Verification items for the finished model (mm, model axes). Give positions to 0.01 mm unless a question says otherwise; leave off trailing zeros. Loops run counter-clockwise (first coordinate to the right, second up) from the corner with the lowest first, then second, coordinate; pieces in that order, holes last. Notation, with made-up numbers: M 24,-25 L 51,-25 A19 ccw 51,-8 Z; hole C -25.5,88.5 d5. An arc over 180 degrees is marked long. Answer in a Markdown table with one row per item.
```python
from build123d import *

# Parameters (mm, degrees)
SKETCH1_W               = 10
SKETCH1_H               = 10
SKETCH1_R               = 2.605
BOSS_EXTRUDE1_DEPTH     = 304.8
CIRPATTERN1_COUNT       = 4
SKETCH2_R               = 6.35
CUT_EXTRUDE1_DEPTH      = 20
CUT_EXTRUDE1_DEPTH_BACK = 30


with BuildPart() as part:
    # Sketch1 → Boss-Extrude1 (new body)
    with BuildSketch(Plane(origin=(0, 0, 0), x_dir=(0, 0, -1), z_dir=(1, 0, 0))):
        Rectangle(SKETCH1_W, SKETCH1_H)
        Circle(SKETCH1_R, mode=Mode.SUBTRACT)
        Polygon((7.474873734, 9.921463197), (2.553410537, 5), (5, 5), (5, 3.203948776), (9.596194078, 7.800142853), align=None)
        Polygon((9.596194078, 3.24), (12.596194078, 3.24), (12.596194078, 12.596194078), (3.24, 12.596194078), (3.24, 9.921463197), (7.474873734, 9.921463197), (9.596194078, 7.800142853), align=None)
    boss_extrude1 = extrude(amount=BOSS_EXTRUDE1_DEPTH)

    # CirPattern1: Boss-Extrude1 ×4 about axis
    cirpattern1_axis = Axis((0, 0, 0), (1, 0, 0))
    for i in range(1, CIRPATTERN1_COUNT):
        add(boss_extrude1.rotate(cirpattern1_axis, i * 360 / CIRPATTERN1_COUNT))

    # Sketch2 → Cut-Extrude1 (cut, two sides)
    with BuildSketch(Plane.XY) as cut_extrude1_sk:
        with Locations((152.4, 0)):
            Circle(SKETCH2_R)
    extrude(amount=CUT_EXTRUDE1_DEPTH, mode=Mode.SUBTRACT)
    extrude(cut_extrude1_sk.sketch, amount=-CUT_EXTRUDE1_DEPTH_BACK, mode=Mode.SUBTRACT)


solid = part.part
```
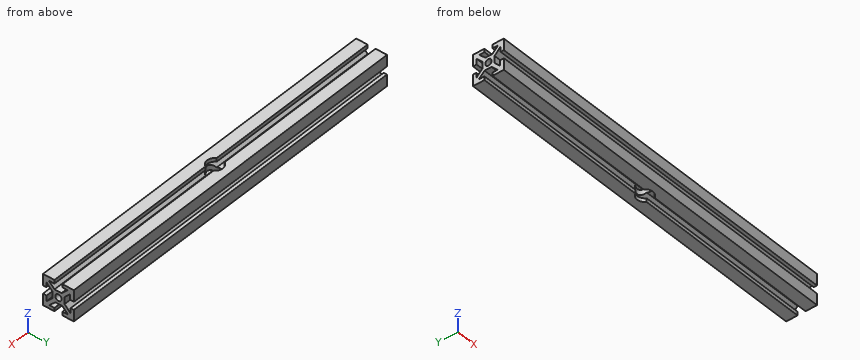
Item 1: Go/stop test with flat-tipped pins: pin 1 (3 mm diameter, centred on x = 103, y = -1.5, fed in from +Z); pin 2 (4.5 mm diameter, centred on x = 88, z = -0.5, fed in from -Y); pin 3 (4 mm diameter, centred on x = 260, y = -0.5, fed in from -Z); pin 4 (4 mm diameter, centred on y = 0, z = 0, fed in from -X) (1 decimal). Record where each tip stops, or that it passes through.
Reported:
| item | result |
|---|---|
| pin 1 | stops at z = 5 |
| pin 2 | stops at y = -5 |
| pin 3 | stops at z = -5 |
| pin 4 | passes through |
Item 2: Scan lines: L1, parallel to Z at x = 161, y = -11; L2, parallel to Z at x = 58, y = -0.25; L3, parallel to X at y = 0, z = 2.75. Record each from-to range of solid material in increasing order. Write a range as [from, to].
Reported:
| item | result |
|---|---|
| L1 | z = [-12.6, -3.24], [3.24, 12.6] |
| L2 | z = [-5, -2.59], [2.59, 5] |
| L3 | x = [0, 146.05], [158.75, 304.8] |
Item 3: Sectioned sample at A-A (y = 0). Record the cut outline in (x, z) (3 decimals), and give its area (3 significant figures).
Reported:
| item | result |
|---|---|
| outline | M 0,-5 L 146.05,-5 L 146.05,-2.605 L 0,-2.605 Z; M 0,2.605 L 146.05,2.605 L 146.05,5 L 0,5 Z; M 158.75,-5 L 304.8,-5 L 304.8,-2.605 L 158.75,-2.605 Z; M 158.75,2.605 L 304.8,2.605 L 304.8,5 L 158.75,5 Z |
| area | 1,400 mm^2 |
Item 4: Sectioned sample at B-B (x = 152.4). State how many separate pieces and enclosed holes the cut face has, and give its area (3 significant figures).
Reported:
| item | result |
|---|---|
| separate pieces | 4 |
| enclosed holes | 0 |
| area | 194 mm^2 |
